For this review, take the finished solid that the model builds, in its own axes (mm). A direction names the side the tool comes from. Round coordinates to 2 decimals unless told otherwise and drop trailing zeros. Order: outer loops, then holes, each group sorted by start corner. A loop starts at its lowest first (then second) coordinate and runs counter-clockwise, first axis right, second up. Notation, with made-up numbers: M 50,-38.5 L 87,-38.5 A10 cw 87,-23.5 Z; hole C -7.5,3.5 d3. An arc over 180 degrees is marked long. Put each result on its own line as item: value.
from build123d import *

# Parameters (mm, degrees)
F0_W          = 23
F0_H          = 17.5
F1_DEPTH      = 10
F2_T          = -1.2
F3_R          = 5.7
F4_DEPTH      = 3
F3_R_2        = 6.7
F5_DEPTH      = 7.5
F6_W          = 6
F6_H          = 2.3
F6_W_2        = 3.5
F6_H_2        = 3.5
F7_DEPTH      = 4
F8_DEPTH      = 6
F10_DEPTH     = 30
F11_T1_DEPTH  = 19
F11_T3_DEPTH  = 26.5
F11_T5_DEPTH  = 13
F11_T7_DEPTH  = 27.7264973081
F11_S11_W     = 2
F11_S11_H     = 2
F11_T12_DEPTH = 2
F11_S17_W     = 2
F11_S17_H     = 2
F11_T18_DEPTH = 2


# Not quite as in the source:
# - a fillet or chamfer that OpenCascade refuses, or shapes differently, is made with other operations: its cross-section is extruded or revolved along the edge and cut away or added


with BuildPart() as f1:
    # F0 (on Front) → F1 (new body)
    with BuildSketch(Plane.XZ):
        Rectangle(F0_W, F0_H)
    extrude(amount=F1_DEPTH)

    # F2
    f2_openings = [f1.faces().sort_by_distance(p)[0] for p in [
        (0, -10, 0),
    ]]
    offset(amount=F2_T, openings=f2_openings)

    # F3 (on face) → F4 (cut)
    with BuildSketch(Plane(origin=(0, 0, 0), x_dir=(-1, 0, 0), z_dir=(0, 1, 0))):
        Circle(F3_R)
    extrude(amount=-F4_DEPTH, mode=Mode.SUBTRACT)

    # F3 (on face) → F5 (join)
    with BuildSketch(Plane(origin=(0, 0, 0), x_dir=(-1, 0, 0), z_dir=(0, 1, 0))):
        Circle(F3_R_2)
        Circle(F3_R, mode=Mode.SUBTRACT)
    extrude(amount=F5_DEPTH)

    # F6 (on face) → F7 (cut)
    with BuildSketch(Plane.XY.offset(8.75)):
        with Locations((1.5, -8.85)):
            Rectangle(F6_W, F6_H)
        with Locations((-5.75, -8.25)):
            Rectangle(F6_W_2, F6_H_2)
    extrude(amount=-F7_DEPTH, mode=Mode.SUBTRACT)

    # F8 (add): a face of the model
    f8_faces = [f1.faces().sort_by_distance(p)[0] for p in [
        (0, -5, -8.75),
    ]]
    extrude(f8_faces, amount=F8_DEPTH)

    # F9 (on face) → F10 (cut)
    with BuildSketch(Plane.YZ.offset(11.5)):
        Polygon((-10, -14.75), (0, -14.75), (-10, -8.9764973081), align=None)
    extrude(amount=-F10_DEPTH, mode=Mode.SUBTRACT)

    # F11: fillet of radius 2 on 7 edges, made by hand

    # F11_s2 → F11_t1 (cut)
    with BuildSketch(Plane.YZ.offset(-9.5)):
        with BuildLine():
            ThreePointArc((0, 6.75), (-0.5857864376, 8.1642135624), (-2, 8.75))
            Line((-2, 8.75), (0, 8.75))
            Line((0, 8.75), (0, 6.75))
        make_face()
    extrude(amount=F11_T1_DEPTH, mode=Mode.SUBTRACT)

    # F11_s4 → F11_t3 (cut)
    with BuildSketch(Plane.XY.offset(-19.75)):
        with BuildLine():
            ThreePointArc((-11.5, -2), (-10.9142135624, -0.5857864376), (-9.5, 0))
            Line((-9.5, 0), (-11.5, 0))
            Line((-11.5, 0), (-11.5, -2))
        make_face()
        with BuildLine():
            ThreePointArc((9.5, 0), (10.9142135624, -0.5857864376), (11.5, -2))
            Line((11.5, -2), (11.5, 0))
            Line((11.5, 0), (9.5, 0))
        make_face()
    extrude(amount=F11_T3_DEPTH, mode=Mode.SUBTRACT)

    # F11_s6 → F11_t5 (cut)
    with BuildSketch(Plane.XZ.offset(2)):
        with BuildLine():
            ThreePointArc((9.5, 8.75), (10.9142135624, 8.1642135624), (11.5, 6.75))
            Line((11.5, 6.75), (11.5, 8.75))
            Line((11.5, 8.75), (9.5, 8.75))
        make_face()
        with BuildLine():
            ThreePointArc((-11.5, 6.75), (-10.9142135624, 8.1642135624), (-9.5, 8.75))
            Line((-9.5, 8.75), (-11.5, 8.75))
            Line((-11.5, 8.75), (-11.5, 6.75))
        make_face()
    extrude(amount=F11_T5_DEPTH, mode=Mode.SUBTRACT)

    # F11_s8 → F11_t7 (cut)
    with BuildSketch(Plane.XY.offset(-13.9764973081)):
        with BuildLine():
            ThreePointArc((-11.5, -8), (-10.9142135624, -9.4142135624), (-9.5, -10))
            Line((-9.5, -10), (-11.5, -10))
            Line((-11.5, -10), (-11.5, -8))
        make_face()
        with BuildLine():
            ThreePointArc((9.5, -10), (10.9142135624, -9.4142135624), (11.5, -8))
            Line((11.5, -8), (11.5, -10))
            Line((11.5, -10), (9.5, -10))
        make_face()
    extrude(amount=F11_T7_DEPTH, mode=Mode.SUBTRACT)


with BuildPart() as f11_tool10:
    # F11_s11 → F11_t12 (new body)
    with BuildSketch(Plane.XZ.offset(2)):
        with Locations((10.5, 7.75)):
            Rectangle(F11_S11_W, F11_S11_H)
    extrude(amount=-F11_T12_DEPTH)

    # F11_s13 → F11_t14 (revolve, cut)
    with BuildSketch(Plane(origin=(9.5, -2, 6.75), x_dir=(-0.7071067812, 0, -0.7071067812), z_dir=(0.7071067812, 0, -0.7071067812))):
        with BuildLine():
            ThreePointArc((0, -2), (2, 0), (0, 2))
            Line((0, 2), (0, -2))
        make_face()
    revolve(axis=Axis((9.5, -2, 6.75), (0, 1, 0)), mode=Mode.SUBTRACT)


with BuildPart() as f1_1:
    add(f1.part)

    # F11_t9: cut F11_tool10
    add(f11_tool10.part, mode=Mode.SUBTRACT)


with BuildPart() as f11_tool16:
    # F11_s17 → F11_t18 (new body)
    with BuildSketch(Plane.YZ.offset(-9.5)):
        with Locations((-1, 7.75)):
            Rectangle(F11_S17_W, F11_S17_H)
    extrude(amount=-F11_T18_DEPTH)

    # F11_s19 → F11_t20 (revolve, cut)
    with BuildSketch(Plane(origin=(-9.5, -2, 6.75), x_dir=(0, -0.7071067812, -0.7071067812), z_dir=(0, 0.7071067812, -0.7071067812))):
        with BuildLine():
            ThreePointArc((0, -2), (2, 0), (0, 2))
            Line((0, 2), (0, -2))
        make_face()
    revolve(axis=Axis((-9.5, -2, 6.75), (-1, 0, 0)), mode=Mode.SUBTRACT)


with BuildPart() as f1_2:
    add(f1_1.part)

    # F11_t15: cut F11_tool16
    add(f11_tool16.part, mode=Mode.SUBTRACT)


solid = f1_2.part
(1) Add section A-A on z = 0. Give the boundary of the cut face in (x, y), then the cut area to 3 significant figures.
A:
outline: M -11.5,-8 A2 ccw -10.3,-9.83 L -10.3,-1.2 L -5.7,-1.2 L -5.7,7.5 L -6.7,7.5 L -6.7,0 L -9.5,0 A2 ccw -11.5,-2 Z; M 5.7,-1.2 L 10.3,-1.2 L 10.3,-9.83 A2 ccw 11.5,-8 L 11.5,-2 A2 ccw 9.5,0 L 6.7,0 L 6.7,7.5 L 5.7,7.5 Z
area: 46.7 mm2
(2) Add section B-B on x = 0. Give the boundary of the cut face in (y, z).
A:
outline: M -10,-8.98 L 0,-14.75 L 0,-6.7 L 7.5,-6.7 L 7.5,-5.7 L -1.2,-5.7 L -1.2,-7.55 L -10,-7.55 Z; M -7.7,7.55 L -1.2,7.55 L -1.2,5.7 L 7.5,5.7 L 7.5,6.7 L 0,6.7 L 0,6.75 A2 ccw -2,8.75 L -7.7,8.75 Z
(3) Add section C-C on y = -5.5. Give the boundary of the cut face in (x, z).
A:
outline: M -11.5,-11.57 L 11.5,-11.57 L 11.5,6.75 A2 ccw 9.5,8.75 L -9.5,8.75 A2 ccw -11.5,6.75 Z; hole M -10.3,-7.55 L 10.3,-7.55 L 10.3,7.55 L -10.3,7.55 Z
(4) To check wall thickness, follow L1, parallel to Z at x = 7.5, y = -2; L2, parallel to X at y = -2, z = -1.5; L3, parallel to Z at x = 0, y = 4.75. State the ranges of each line that lie inside material, in increasing order.
A:
L1: z = -13.6 to -7.55, 7.55 to 8.75
L2: x = -11.5 to -10.3, 10.3 to 11.5
L3: z = -6.7 to -5.7, 5.7 to 6.7
(5) For faces 4 (the face through (0, -5, 7.55)), 5 (the face through (-1.5, -9, 8)), 6 (the face through (6.694, 3.698, 0.295)), 7 (the face through (-3, -10, 8)), list the 3-axis set-ups (+Z, -Z, +X, -X, +Y, -Y) from which the entire face can be reached by the end or side of a thin tool; tool diameter is ignored.
A:
face 4: -Y
face 5: +Z, -Y
face 6: +Y
face 7: +Z, -Z, +X, -X, -Y
(6) Add section D-D on x = -8.75. Give the boundary of the cut face in (y, z).
A:
outline: M -10,-8.98 L 0,-14.75 L 0,6.75 A2 ccw -2,8.75 L -10,8.75 L -10,7.55 L -1.2,7.55 L -1.2,-7.55 L -10,-7.55 Z
(7) Insertion check: pin 1 Ø6 at (y, z) = (3.5, -2.5) entering from +X; pin 2 Ø1.3 at (y, z) = (-8.5, 8) entering from -X; pin 3 Ø7.5 at (x, z) = (3, 3) entering from -Y. Each pin has a flat end and moves straight along its axis. Give the tip position at first contact, or say it passes through.
A:
pin 1: stops at x = 6.7
pin 2: stops at x = -11.41
pin 3: stops at y = -1.2
(8) Draft analysis for pull direction X (two halves, no side actions). For faces 1 (the face through (0, 0, -9)), 2 (the face through (10.9, -0.57, -4.15)), 3 (the face through (-6, -6.5, 8)), state which applies: released by +X, released by -X, zero draft, split by the parting line, or undercut.
A:
face 1: zero draft
face 2: released by +X
face 3: undercut
